Part print with two shaded views. Sizes in mm from the minimum x, y, z corner. Coordinates: 2 decimals unless noted, no trailing zeros. Write each loop counter-clockwise with the first axis right and the second up, starting at its lowest first coordinate (ties: lowest second). Pieces come first, ordered by that corner, then holes.
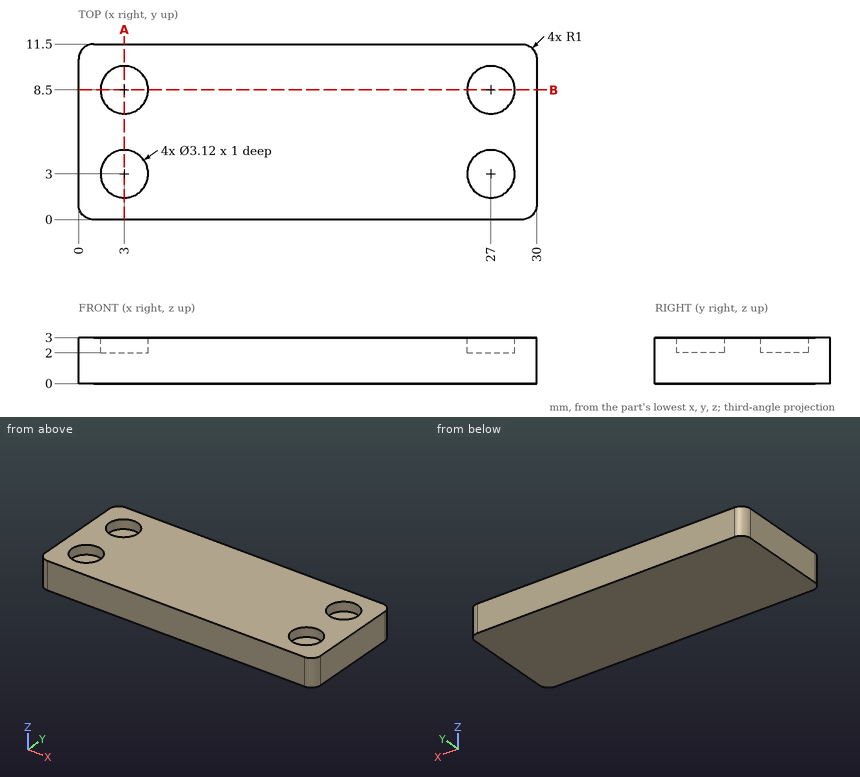
(1) Probe L1, parallel to Y at x = 3, z = 2.4; L2, parallel to X at y = 8.5, z = 2.75; L3, parallel to Y at x = 28, z = 2.35 (1 decimal). List the from-to ranges inside material, lowest first.
(2) Slice it at B-B, the plane y = 8.5. List the corners of the cut face in (x, z).
(3) Slice it at A-A, the plane x = 3. List the corners of the cut face in (y, z).
(4) Flat gauge pin, fed straight in: P1, Ø0.9, axis at x = 26.5, y = 3.5, coming from the +Z side. Where does the tip first touch, or does it go through?
Results:
1. L1: y = 0 to 1.44, 4.56 to 6.94, 10.06 to 11.5
1. L2: x = 0 to 1.44, 4.56 to 25.44, 28.56 to 30
1. L3: y = 0 to 1.8, 4.2 to 7.3, 9.7 to 11.5
2. outline: (0, 0) - (30, 0) - (30, 3) - (28.56, 3) - (28.56, 2) - (25.44, 2) - (25.44, 3) - (4.56, 3) - (4.56, 2) - (1.44, 2) - (1.44, 3) - (0, 3) - close
3. outline: (0, 0) - (11.5, 0) - (11.5, 3) - (10.06, 3) - (10.06, 2) - (6.94, 2) - (6.94, 3) - (4.56, 3) - (4.56, 2) - (1.44, 2) - (1.44, 3) - (0, 3) - close
4. P1: stops at z = 2
